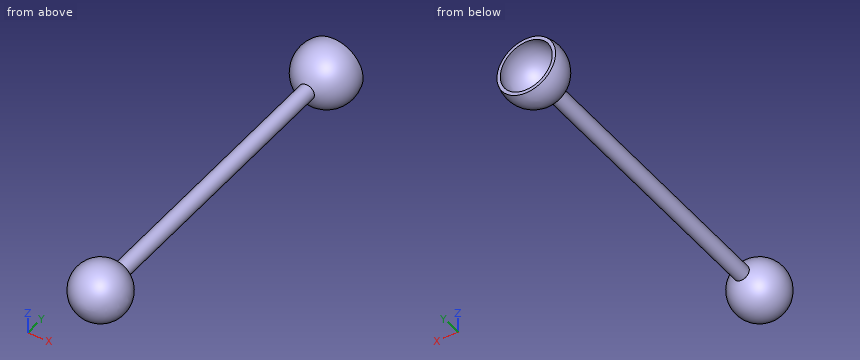
```python
from build123d import *

# Parameters (mm, degrees)
BOSS_EXTRUDE1_REACH             = 24.045
BOSS_EXTRUDE1_END_RADIUS        = 9
SKETCH3_R                       = 2.5
BOSS_EXTRUDE1_DIRECTION_2_DEPTH = 100
CUT_EXTRUDE1_DEPTH              = 10
CUT_EXTRUDE1_DEPTH_BACK         = 10
SKETCH5_W                       = 20
SKETCH5_H                       = 8.579104118


# Read off the part's stored shape, not the designer's step: Shell1
with BuildPart() as part:
    # Sketch1 → Revolve1 (revolve)
    with BuildSketch(Plane.XY):
        with BuildLine():
            Line((0, -9), (0, 9))
            ThreePointArc((0, 9), (9, 0), (0, -9))
        make_face()
    revolve(axis=Axis((0, -9, 0), (0, 1, 0)))

    # Boss-Extrude1: up to this sphere (the profile starts outside it)
    boss_extrude1_end = Location((0, 0, 0)) * Sphere(BOSS_EXTRUDE1_END_RADIUS, mode=Mode.PRIVATE)
    # Sketch3 → Boss-Extrude1 (add, up to the surface)
    with BuildSketch(Plane(origin=(0, 9, 0), x_dir=(1, 0, 0), z_dir=(0, 1, 0)), mode=Mode.PRIVATE) as boss_extrude1_sk1:
        with Locations(Location((0, 0, 0), (0, 0, 90))):
            Circle(SKETCH3_R)
    boss_extrude1_tool1 = extrude(boss_extrude1_sk1.sketch, amount=-BOSS_EXTRUDE1_REACH, mode=Mode.PRIVATE) - boss_extrude1_end
    add(boss_extrude1_tool1.solids().sort_by_distance((0, 9, 0))[0])

    # Sketch3 → Boss-Extrude1 direction 2 (add)
    with BuildSketch(Plane(origin=(0, 9, 0), x_dir=(1, 0, 0), z_dir=(0, 1, 0))):
        with Locations(Location((0, 0, 0), (0, 0, 90))):
            Circle(SKETCH3_R)
    extrude(amount=BOSS_EXTRUDE1_DIRECTION_2_DEPTH)

    # Sketch4 → Revolve2 (revolve)
    with BuildSketch(Plane(origin=(0, 0, 0), x_dir=(0, 0, -1), z_dir=(1, 0, 0))):
        with BuildLine():
            Line((0, 109), (0, 99))
            ThreePointArc((0, 99), (10, 109), (0, 119))
            Line((0, 119), (0, 109))
        make_face()
    revolve(axis=Axis((0, 109, 0), (0, 1, 0)))

    # Sketch5 → Cut-Extrude1 (cut, two sides: drawn at the far end of the back side and taken through both)
    with BuildSketch(Plane(origin=(0, 0, 0), x_dir=(0, 0, -1), z_dir=(1, 0, 0)).offset(-CUT_EXTRUDE1_DEPTH_BACK)):
        with Locations((0, 116.710447941)):
            Rectangle(SKETCH5_W, SKETCH5_H)
    extrude(amount=CUT_EXTRUDE1_DEPTH + CUT_EXTRUDE1_DEPTH_BACK, mode=Mode.SUBTRACT)

    # Shell1 outline → Shell1 (revolve, cut)
    with BuildSketch(Plane.XY):
        with BuildLine():
            Line((0, 112.42089589), (0, 100))
            ThreePointArc((0, 100), (7.476231103, 103.989414356), (8.324510274, 112.42089589))
            Line((8.324510274, 112.42089589), (0, 112.42089589))
        make_face()
    revolve(axis=Axis((0, 0, 0), (0, 1, 0)), mode=Mode.SUBTRACT)


solid = part.part
```
Model file for the job. Use its own axes, mm. Give positions to 0.01 mm unless a question says otherwise; leave off trailing zeros. Write each loop counter-clockwise with the first axis right and the second up, starting at its lowest first coordinate (ties: lowest second). Pieces come first, ordered by that corner, then holes. Notation, with made-up numbers: (-21, -29) - (23, -29) arc R15 ccw to (23, -22) - close; hole circle Ø1 at (54.25, 50.5). An arc over 180 degrees is marked (long way). One line per question, with ' | ' between items. Start each with the question number.
(1) Slice it at C-C on y = 58.5. Write the cut outline in (x, z).
(2) Pin check, flat tips, straight feed: P1, Ø2, axis at x = 4, z = 2, coming from the -Y side; P2, Ø1, axis at x = -1, z = -0.5, coming from the +Y side; P3, Ø5, axis at x = -1, z = 3.5, coming from the +Y side; P4, Ø5, axis at x = -5, z = -5, coming from the +Y side. Stop position of each tip, or through.
(3) Slice it at D-D on x = 0. Write the cut outline in (y, z), plus the area to 3 significant figures.
(4) Slice it at A-A on z = 3.5. Write the cut outline in (x, y) (1 decimal).
(5) Slice it at B-B on x = -5.5. Write the cut outline in (y, z), plus the area to 3 significant figures.
(6) Wall check: line 1 along X through (y, z) = (63, -0.25); line 2 along Y through (x, z) = (-6.5, -1.5); line 3 along Y through (x, z) = (4.5, 1.5). Give the ranges that are in metal, low to high. Write a range as from..to.
Results below:
1) outline: circle Ø5 at (0, 0)
2) P1: y = -8.3 | P2: y = 100.15 | P3: y = 102.42 | P4: y = 112.42
3) outline: (8.65, -2.5) - (99.32, -2.5) arc R10 ccw to (112.42, -9.4) - (112.42, -8.32) arc R9 cw (long way) to (112.42, 8.32) - (112.42, 9.4) arc R10 ccw to (99.32, 2.5) - (8.65, 2.5) arc R9 ccw (long way) to start | area: 742 mm^2
4) outline: (-8.7, 112.4) arc R9.4 ccw (long way) to (8.7, 112.4) - (7.6, 112.4) arc R8.3 cw (long way) to (-7.6, 112.4) - close; circle Ø16.6 at (0, 0)
5) outline: circle Ø14.25 at (0, 0); (112.42, -7.62) - (112.42, -6.25) arc R7.12 cw (long way) to (112.42, 6.25) - (112.42, 7.62) arc R8.35 ccw (long way) to start | area: 198 mm^2
6) line 1: -2.49..2.49 | line 2: -6.04..6.04, 101.55..102.96 | line 3: -7.65..7.65, 100.2..101.35
